Can you work these out from the model? Positions are in its coordinate system, mm. A direction names the side the tool comes from. Round coordinates to 2 decimals unless told otherwise and drop trailing zeros. Order: outer loops, then holes, each group sorted by start corner. A loop starts at its lowest first (then second) coordinate and runs counter-clockwise, first axis right, second up.
Q1. We'd pull the mould along Y, two halves only. Please class faces 1 (the face through (15.875, 76, -9)), 2 (the face through (25.4, 5, -77)), 3 (the face through (123.38, 123.18, -77.09)): pulls with the +Y half, pulls with the -Y half, needs draft (parallel to the pull), parting line crosses it, or undercut.
Q2. If we section it at A-A (z = -78.5): Please give me the cut outline in (x, y) (1 decimal).
Q3. If I drill on line 1 (Z direction, x = 42.5, y = 59); line 2 (Y direction, x = 44.5, z = -112.5) (3 decimals); line 3 (Y direction, x = 27, z = -14), over which ranges is the centre line in solid material (lowest first)?
Q4. If we section it at C-C (y = 44): Please give me the cut outline in (x, z), plus the area to 3 significant figures.
Q5. Will these pins go through, and if not, where does the flat tip stop? P1, Ø5, axis at y = 66, z = -2.5, coming from the +X side; P2, Ø12, axis at y = 23, z = -107, coming from the -X side; P3, Ø6.5, axis at x = 19, z = -8, coming from the -Y side.
Q6. If we section it at B-B (x = 38.1): Count the separate pieces of the cut face and the enclosed holes in it, plus the area to 3 significant figures.
Q7. For faces 4 (the face through (123.38, 3.82, -77.09)), 5 (the face through (25.4, 63, -3)), 6 (the face through (56, 12.7, -77)), 7 (the face through (57.95, 123.18, -148.78)), 8 (the face through (39.99, 62.05, -146.14)), which set-ups out of +Z, -Z, +X, -X, +Y, -Y let a thin tool reach every point of the face, with its end or its side?
from build123d import *

# Parameters (mm, degrees)
SKETCH1_W           = 127
SKETCH1_H           = 152.4
BOSS_EXTRUDE1_DEPTH = 127
SHELL1_T            = -12.7
FILLET1_R           = 12.7
SKETCH3_W           = 23.988888889
SKETCH3_H           = 69.85
CUT_EXTRUDE1_DEPTH  = 9.525
SKETCH4_W           = 34.925
SKETCH4_H           = 79.375
CUT_EXTRUDE2_DEPTH  = 3.175
SKETCH5_W           = 12.7
SKETCH5_H           = 28.575
CUT_EXTRUDE3_DEPTH  = 6.35
CUT_EXTRUDE4_REACH  = 233.492
SKETCH6_W           = 6.35
SKETCH6_H           = 3.81
SKETCH7_R           = 7.9375
CUT_EXTRUDE5_DEPTH  = 11.1125
CUT_EXTRUDE6_REACH  = 231.749
SKETCH8_W           = 46.0375
SKETCH8_H           = 20.6375
CUT_EXTRUDE7_REACH  = 237.55
SKETCH9_R           = 2.38125
CUT_EXTRUDE8_REACH  = 237.55


with BuildPart() as part:
    # Sketch1 → Boss-Extrude1 (new body)
    with BuildSketch(Plane(origin=(0, 0, 0), x_dir=(1, 0, 0), z_dir=(0, 1, 0))):
        with Locations((63.5, 76.2)):
            Rectangle(SKETCH1_W, SKETCH1_H)
    extrude(amount=BOSS_EXTRUDE1_DEPTH)

    # Shell1
    shell1_openings = [part.faces().sort_by_distance(p)[0] for p in [
        (0, 63.5, -76.2),
    ]]
    offset(amount=SHELL1_T, openings=shell1_openings, kind=Kind.INTERSECTION)

    # Fillet1
    fillet1_edges = [part.edges().sort_by_distance(p)[0] for p in [
        (127, 127, -76.2),
        (63.5, 127, -152.4),
        (63.5, 0, -152.4),
        (127, 0, -76.2),
        (63.5, 0, 0),
        (63.5, 127, 0),
        (127, 63.5, -152.4),
        (127, 63.5, 0),
    ]]
    fillet(fillet1_edges, radius=FILLET1_R)

    # Sketch3 → Cut-Extrude1 (cut)
    with BuildSketch(Plane.XZ):
        with Locations((37.394444445, -76.2)):
            Rectangle(SKETCH3_W, SKETCH3_H)
    extrude(amount=-CUT_EXTRUDE1_DEPTH, mode=Mode.SUBTRACT)

    # Sketch4 → Cut-Extrude2 (cut)
    with BuildSketch(Plane(origin=(0, 12.7, 0), x_dir=(1, 0, 0), z_dir=(0, 1, 0))):
        with Locations((37.39388, 76.2)):
            Rectangle(SKETCH4_W, SKETCH4_H)
    extrude(amount=-CUT_EXTRUDE2_DEPTH, mode=Mode.SUBTRACT)

    # Sketch5 → Cut-Extrude3 (cut)
    with BuildSketch(Plane.XY):
        with Locations((19.05, 63.5)):
            Rectangle(SKETCH5_W, SKETCH5_H)
    extrude(amount=-CUT_EXTRUDE3_DEPTH, mode=Mode.SUBTRACT)

    # Sketch6 → Cut-Extrude4 (cut, up to next)
    with BuildSketch(Plane.XY.offset(-6.35), mode=Mode.PRIVATE) as cut_extrude4_sk1:
        with Locations((19.05, 75.8825)):
            Rectangle(SKETCH6_W, SKETCH6_H)
    cut_extrude4_tool1 = extrude(cut_extrude4_sk1.sketch, amount=-CUT_EXTRUDE4_REACH, mode=Mode.PRIVATE) & part.part
    add(cut_extrude4_tool1.solids().sort_by_distance((19.05, 75.8825, -6.35))[0], mode=Mode.SUBTRACT)

    # Sketch7 → Cut-Extrude5 (cut)
    with BuildSketch(Plane(origin=(127, 0, 0), x_dir=(0, 0, -1), z_dir=(1, 0, 0))):
        with Locations((63.5, 63.5)):
            Circle(SKETCH7_R)
        with Locations((88.9, 63.5)):
            Circle(SKETCH7_R)
    extrude(amount=-CUT_EXTRUDE5_DEPTH, mode=Mode.SUBTRACT)

    # Sketch8 → Cut-Extrude6 (cut, up to next)
    with BuildSketch(Plane(origin=(115.8875, 0, 0), x_dir=(0, 0, -1), z_dir=(1, 0, 0)), mode=Mode.PRIVATE) as cut_extrude6_sk1:
        with Locations((76.2, 63.5)):
            Rectangle(SKETCH8_W, SKETCH8_H)
    cut_extrude6_tool1 = extrude(cut_extrude6_sk1.sketch, amount=-CUT_EXTRUDE6_REACH, mode=Mode.PRIVATE) & part.part
    add(cut_extrude6_tool1.solids().sort_by_distance((115.8875, 63.5, -76.2))[0], mode=Mode.SUBTRACT)

    # Sketch9 → Cut-Extrude7 (cut, up to next)
    with BuildSketch(Plane(origin=(0, 0, -152.4), x_dir=(-1, 0, 0), z_dir=(0, 0, -1)), mode=Mode.PRIVATE) as cut_extrude7_sk1:
        with Locations((-38.1, 76.2)):
            Circle(SKETCH9_R)
    cut_extrude7_tool1 = extrude(cut_extrude7_sk1.sketch, amount=-CUT_EXTRUDE7_REACH, mode=Mode.PRIVATE) & part.part
    # Sketch9 → Cut-Extrude7 (cut, up to next)
    with BuildSketch(Plane(origin=(0, 0, -152.4), x_dir=(-1, 0, 0), z_dir=(0, 0, -1)), mode=Mode.PRIVATE) as cut_extrude7_sk2:
        with Locations((-38.1, 63.5)):
            Circle(SKETCH9_R)
    cut_extrude7_tool2 = extrude(cut_extrude7_sk2.sketch, amount=-CUT_EXTRUDE7_REACH, mode=Mode.PRIVATE) & part.part
    # Sketch9 → Cut-Extrude7 (cut, up to next)
    with BuildSketch(Plane(origin=(0, 0, -152.4), x_dir=(-1, 0, 0), z_dir=(0, 0, -1)), mode=Mode.PRIVATE) as cut_extrude7_sk3:
        with Locations((-38.1, 50.8)):
            Circle(SKETCH9_R)
    cut_extrude7_tool3 = extrude(cut_extrude7_sk3.sketch, amount=-CUT_EXTRUDE7_REACH, mode=Mode.PRIVATE) & part.part
    add(cut_extrude7_tool1.solids().sort_by_distance((38.1, 76.2, -152.4))[0], mode=Mode.SUBTRACT)
    add(cut_extrude7_tool2.solids().sort_by_distance((38.1, 63.5, -152.4))[0], mode=Mode.SUBTRACT)
    add(cut_extrude7_tool3.solids().sort_by_distance((38.1, 50.8, -152.4))[0], mode=Mode.SUBTRACT)

    # Sketch10 → Cut-Extrude8 (cut, up to next)
    with BuildSketch(Plane(origin=(0, 127, 0), x_dir=(1, 0, 0), z_dir=(0, 1, 0)), mode=Mode.PRIVATE) as cut_extrude8_sk1:
        with BuildLine():
            Line((61.9125, 88.9), (61.9125, 85.725))
            ThreePointArc((61.9125, 85.725), (63.5, 84.1375), (65.0875, 85.725))
            Line((65.0875, 85.725), (65.0875, 88.9))
            ThreePointArc((65.0875, 88.9), (63.5, 90.4875), (61.9125, 88.9))
        make_face()
    cut_extrude8_tool1 = extrude(cut_extrude8_sk1.sketch, amount=-CUT_EXTRUDE8_REACH, mode=Mode.PRIVATE) & part.part
    # Sketch10 → Cut-Extrude8 (cut, up to next)
    with BuildSketch(Plane(origin=(0, 127, 0), x_dir=(1, 0, 0), z_dir=(0, 1, 0)), mode=Mode.PRIVATE) as cut_extrude8_sk2:
        with BuildLine():
            Line((61.9125, 66.675), (61.9125, 63.5))
            ThreePointArc((61.9125, 63.5), (63.5, 61.9125), (65.0875, 63.5))
            Line((65.0875, 63.5), (65.0875, 66.675))
            ThreePointArc((65.0875, 66.675), (63.5, 68.2625), (61.9125, 66.675))
        make_face()
    cut_extrude8_tool2 = extrude(cut_extrude8_sk2.sketch, amount=-CUT_EXTRUDE8_REACH, mode=Mode.PRIVATE) & part.part
    add(cut_extrude8_tool1.solids().sort_by_distance((63.5, 127, -87.3125))[0], mode=Mode.SUBTRACT)
    add(cut_extrude8_tool2.solids().sort_by_distance((63.5, 127, -65.0875))[0], mode=Mode.SUBTRACT)


solid = part.part
Solution:
1. face 1: undercut
1. face 2: needs draft
1. face 3: pulls with the +Y half
2. outline: (0, 0) - (25.4, 0) - (25.4, 9.5) - (19.9, 9.5) - (19.9, 12.7) - (0, 12.7) - close; (0, 114.3) - (114.3, 114.3) - (114.3, 73.8) - (115.9, 73.8) - (115.9, 53.2) - (114.3, 53.2) - (114.3, 12.7) - (54.9, 12.7) - (54.9, 9.5) - (49.4, 9.5) - (49.4, 0) - (114.3, 0) arc R12.7 ccw to (127, 12.7) - (127, 114.3) arc R12.7 ccw to (114.3, 127) - (0, 127) - close
3. line 1: z = -152.4 to -139.7, -12.7 to 0
3. line 2: y = 0 to 9.525, 114.3 to 127
3. line 3: y = 0 to 12.7, 114.3 to 127
4. outline: (0, -152.4) - (114.3, -152.4) arc R12.7 ccw to (127, -139.7) - (127, -12.7) arc R12.7 ccw to (114.3, 0) - (0, 0) - (0, -12.7) - (114.3, -12.7) - (114.3, -139.7) - (0, -139.7) - close
4. area: 4,770 mm2
5. P1: stops at x = 124.4
5. P2: stops at x = 114.3
5. P3: stops at y = 0.08
6. separate pieces: 4
6. enclosed holes: 0
6. area: 5,210 mm2
7. face 4: +Z, -Z, +X, -Y
7. face 5: +Z
7. face 6: -X
7. face 7: -Z, +X, -X, +Y
7. face 8: -Z
